Geometry: final body of the model. Coordinates: model frame, mm. A direction names the side the tool comes from. Give positions to 0.01 mm unless a question says otherwise; leave off trailing zeros. Write each loop counter-clockwise with the first axis right and the second up, starting at its lowest first coordinate (ties: lowest second). Pieces come first, ordered by that corner, then holes. Notation, with made-up numbers: (44, -31) -> (56, -31) arc R12 ccw to (56, -13) -> close; hole circle Ø11 at (49.25, 77.5). An arc over 180 degrees is marked (long way). Answer as a JSON object with one key per item and string values. Group by question number.
(1) Material intervals for probe 1 along Z at (x, y) = (3.8, 0); probe 2 along Z at (x, y) = (3.9, 16); probe 3 along Y at (x, z) = (4.1, 13), sorted ascending.
(2) Section query D-D on y = 12. Output: boundary loops of the cut face in (x, z).
(3) Set-up query: faces 4 (the face through (0, 10, 13)), 5 (the face through (0, 9, 17)), 6 (the face through (2.75, 0, -11)), 7 (the face through (0, 4, -1)). Return all of +Z, -Z, +X, -X, +Y, -Y with unobstructed straight access to the full face (end or side cutting, diameter ignored); none if empty.
(4) Section query C-C on x = 6.25. Output: boundary loops of the cut face in (y, z), plus the area to 3 significant figures.
(5) Section query A-A on z = 13. Output: boundary loops of the cut face in (x, y).
(6) Section query B-B on z = -7.5. Output: boundary loops of the cut face in (x, y), plus the area to 3 significant figures.
(7) Draft query along Z for faces 1 (the face through (5.09, 0.07, -13.5)), 2 (the face through (5, 0, 45)), 3 (the face through (-2.75, 0, -11)). Return one class per face: +Z half, -Z half, draft (parallel to the pull), parting line (faces both ways), or undercut.
(8) Contact query for flat-ended pins moving along their axis: pin 1 Ø4 at (x, y) = (-0.5, 1) entering from +Z; pin 2 Ø1.8 at (x, y) = (0, 1.5) entering from -Z; pin 3 Ø1 at (x, y) = (3, 1.5) entering from +Z; pin 4 Ø2.5 at (y, z) = (16, 13) entering from +X. Output: stop coordinate, or through.
from build123d import *

# Parameters (mm, degrees)
CROQUIS1_R              = 1.5
SALIENTE_EXTRUIR1_DEPTH = 7.5
CROQUIS2_W              = 8
CROQUIS2_H              = 10
CROQUIS2_W_2            = 16
CROQUIS2_H_2            = 8
CROQUIS2_W_3            = 10
CORTAR_EXTRUIR1_DEPTH   = 2.75
REDONDEO1_R             = 1


with BuildPart() as part:
    # Croquis1 → Saliente-Extruir1 (new, symmetric)
    with BuildSketch(Plane(origin=(0, 0, 0), x_dir=(0, 0, -1), z_dir=(1, 0, 0))):
        with BuildLine():
            Line((-15, -4), (15, -4))
            ThreePointArc((15, -4), (19, 0), (15, 4))
            Line((15, 4), (-9, 4))
            Line((-9, 4), (-9, 16))
            ThreePointArc((-9, 16), (-13, 20), (-17, 16))
            Line((-17, 16), (-17, 4))
            Line((-17, 4), (-41, 4))
            ThreePointArc((-41, 4), (-45, 0), (-41, -4))
            Line((-41, -4), (-15, -4))
        make_face()
        with Locations((15, 0)):
            Circle(CROQUIS1_R, mode=Mode.SUBTRACT)
        with Locations((-13, 16)):
            Circle(CROQUIS1_R, mode=Mode.SUBTRACT)
        with Locations((-41, 0)):
            Circle(CROQUIS1_R, mode=Mode.SUBTRACT)
    extrude(amount=SALIENTE_EXTRUIR1_DEPTH, both=True)

    # Croquis2 → Cortar-Extruir1 (cut, symmetric)
    with BuildSketch(Plane(origin=(0, 0, 0), x_dir=(0, 0, -1), z_dir=(1, 0, 0))):
        with Locations((-13, 15)):
            Rectangle(CROQUIS2_W, CROQUIS2_H)
        with Locations((11, 0)):
            Rectangle(CROQUIS2_W_2, CROQUIS2_H_2)
        with Locations((-40, 0)):
            Rectangle(CROQUIS2_W_3, CROQUIS2_H_2)
    extrude(amount=CORTAR_EXTRUIR1_DEPTH, both=True, mode=Mode.SUBTRACT)

    # Redondeo1
    redondeo1_edges = [part.edges().sort_by_distance(p)[0] for p in [
        (2.75, 10, 13),
        (-2.75, 10, 13),
        (2.75, 0, 35),
        (-2.75, 0, 35),
        (2.75, 0, -3),
        (-2.75, 0, -3),
    ]]
    fillet(redondeo1_edges, radius=REDONDEO1_R)


solid = part.part
Answer list:
{
 "1": {"probe 1": "-19 to -16.5, -13.5 to 39.5, 42.5 to 45", "probe 2": "9 to 11.5, 14.5 to 17", "probe 3": "-4 to 14.5, 17.5 to 20"},
 "2": {"outline": "(-7.5, 9) -> (-2.75, 9) -> (-2.75, 17) -> (-7.5, 17) -> close; (2.75, 9) -> (7.5, 9) -> (7.5, 17) -> (2.75, 17) -> close"},
 "3": {"face 4": "+Z, -Z, +Y", "face 5": "+Z, +X, -X, +Y", "face 6": "-Z, +Y, -Y", "face 7": "-Z, +X, -X, +Y"},
 "4": {"outline": "(-4, -15) arc R4 ccw to (4, -15) -> (4, 9) -> (16, 9) arc R4 ccw to (16, 17) -> (4, 17) -> (4, 41) arc R4 ccw to (-4, 41) -> close; hole circle Ø3 at (0, -15); hole circle Ø3 at (0, 41); hole circle Ø3 at (16, 13)", "area": "598 mm2"},
 "5": {"outline": "(-7.5, -4) -> (7.5, -4) -> (7.5, 14.5) -> (2.75, 14.5) -> (2.75, 11) arc R1 cw to (1.75, 10) -> (-1.75, 10) arc R1 cw to (-2.75, 11) -> (-2.75, 14.5) -> (-7.5, 14.5) -> close; (-7.5, 17.5) -> (-2.75, 17.5) -> (-2.75, 20) -> (-7.5, 20) -> close; (2.75, 17.5) -> (7.5, 17.5) -> (7.5, 20) -> (2.75, 20) -> close"},
 "6": {"outline": "(-7.5, -4) -> (-2.75, -4) -> (-2.75, 4) -> (-7.5, 4) -> close; (2.75, -4) -> (7.5, -4) -> (7.5, 4) -> (2.75, 4) -> close", "area": "76.0 mm2"},
 "7": {"face 1": "undercut", "face 2": "+Z half", "face 3": "draft"},
 "8": {"pin 1": "z = 35.34", "pin 2": "z = -3", "pin 3": "z = 44.87", "pin 4": "through"}
}
